from build123d import *

# Parameters (mm, degrees)
SALIENTE_EXTRUIR1_DEPTH    = 2
CROQUIS3_W                 = 28.5
CROQUIS3_H                 = 54
SALIENTE_EXTRUIR2_DEPTH    = 21
CORTAR_EXTRUIR2_DEPTH      = 21
CORTAR_EXTRUIR2_DEPTH_BACK = 61
CORTAR_EXTRUIR2_START      = -23
CROQUIS7_W                 = 26.5
CROQUIS7_H                 = 52
CROQUIS10_W                = 18.5
CROQUIS10_H                = 13
CORTAR_EXTRUIR3_DEPTH      = 10
CROQUIS11_W                = 28.5
CROQUIS11_H                = 54
CORTAR_EXTRUIR4_DEPTH      = 0.9
CROQUIS12_W                = 30
CROQUIS12_H                = 30
CORTAR_EXTRUIR6_DEPTH      = 20.6
CROQUIS13_W                = 3
CROQUIS13_H                = 16
SALIENTE_EXTRUIR5_DEPTH    = 6
SALIENTE_EXTRUIR9_DEPTH    = 16
SALIENTE_EXTRUIR10_DEPTH   = 16
SALIENTE_EXTRUIR11_DEPTH   = 16
SALIENTE_EXTRUIR12_DEPTH   = 16
CROQUIS25_W                = 4.5
CROQUIS25_H                = 1.45
CORTAR_EXTRUIR7_DEPTH      = 0.9
CORTAR_EXTRUIR9_DEPTH      = 0.9
CORTAR_EXTRUIR9_DEPTH_BACK = 1
CROQUIS26_W                = 6
CROQUIS26_H                = 5
CROQUIS32_R                = 2.5
SALIENTE_EXTRUIR13_DEPTH   = 29
CROQUIS36_R                = 1
CORTAR_EXTRUIR10_DEPTH     = 4.5
CROQUIS39_R                = 1
CORTAR_EXTRUIR11_DEPTH     = 4.5
CROQUIS38_R                = 1
CORTAR_EXTRUIR12_DEPTH     = 4.5
CROQUIS37_R                = 1
CORTAR_EXTRUIR13_DEPTH     = 4.5


with BuildPart() as part:
    # Croquis1 → Saliente-Extruir1 (new body)
    with BuildSketch(Plane(origin=(0, 0, 0), x_dir=(1, 0, 0), z_dir=(0, 1, 0))):
        with BuildLine():
            Line((-76.52774776, -47.188914739), (-76.52774776, 21.977990865))
            ThreePointArc((-76.52774776, 21.977990865), (-51.168030611, 47.337708015), (-25.808313462, 21.977990865))
            Line((-25.808313462, 21.977990865), (-25.808313462, -47.033075243))
            ThreePointArc((-25.808313462, -47.033075243), (-51.106035712, -67.287819919), (-76.52774776, -47.188914739))
        make_face()
    extrude(amount=SALIENTE_EXTRUIR1_DEPTH)

    # Croquis3 → Saliente-Extruir2 (add)
    with BuildSketch(Plane(origin=(0, 2, 0), x_dir=(1, 0, 0), z_dir=(0, 1, 0))):
        with Locations((-51.124943413, -32.32840731)):
            Rectangle(CROQUIS3_W, CROQUIS3_H)
    extrude(amount=SALIENTE_EXTRUIR2_DEPTH)

    # Croquis7 → Cortar-Extruir2 (cut, two sides: drawn at the far end of the back side and taken through both)
    with BuildSketch(Plane(origin=(0, 23, 0), x_dir=(1, 0, 0), z_dir=(0, 1, 0)).offset(CORTAR_EXTRUIR2_START - CORTAR_EXTRUIR2_DEPTH_BACK)):
        with Locations((-51.124943413, -32.32840731)):
            Rectangle(CROQUIS7_W, CROQUIS7_H)
    extrude(amount=CORTAR_EXTRUIR2_DEPTH + CORTAR_EXTRUIR2_DEPTH_BACK, mode=Mode.SUBTRACT)

    # Croquis10 → Cortar-Extruir3 (cut)
    with BuildSketch(Plane(origin=(0, 0, 5.32840731), x_dir=(-1, 0, 0), z_dir=(0, 0, -1))):
        with Locations((51.124943413, 8.5)):
            Rectangle(CROQUIS10_W, CROQUIS10_H)
    extrude(amount=-CORTAR_EXTRUIR3_DEPTH, mode=Mode.SUBTRACT)

    # Croquis11 → Cortar-Extruir4 (cut)
    with BuildSketch(Plane.XZ):
        with Locations((-51.124943413, 32.32840731)):
            Rectangle(CROQUIS11_W, CROQUIS11_H)
    extrude(amount=-CORTAR_EXTRUIR4_DEPTH, mode=Mode.SUBTRACT)

    # Croquis12 → Cortar-Extruir6 (cut)
    with BuildSketch(Plane(origin=(0, 2, 0), x_dir=(1, 0, 0), z_dir=(0, 1, 0))):
        with Locations((-51.168030611, 16.67159269)):
            Rectangle(CROQUIS12_W, CROQUIS12_H)
    extrude(amount=-CORTAR_EXTRUIR6_DEPTH, mode=Mode.SUBTRACT)

    # Croquis13 → Saliente-Extruir5 (add)
    with BuildSketch(Plane(origin=(0, 2, 0), x_dir=(1, 0, 0), z_dir=(0, 1, 0))):
        with Locations((-29.308313462, -38.804003852)):
            Rectangle(CROQUIS13_W, CROQUIS13_H)
        with Locations((-73.02774776, -38.95348914)):
            Rectangle(CROQUIS13_W, CROQUIS13_H)
        with Locations((-73.02774776, 13.977990865)):
            Rectangle(CROQUIS13_W, CROQUIS13_H)
        with Locations((-29.308313462, 13.977990865)):
            Rectangle(CROQUIS13_W, CROQUIS13_H)
    extrude(amount=SALIENTE_EXTRUIR5_DEPTH)

    # Croquis18 → Saliente-Extruir9 (add)
    with BuildSketch(Plane.XY.offset(46.804003852)):
        Polygon((-27.808313462, 8), (-27.808313462, 5.3), (-26.608313462, 5.3), align=None)
    extrude(amount=-SALIENTE_EXTRUIR9_DEPTH)

    # Croquis21 → Saliente-Extruir10 (add)
    with BuildSketch(Plane.XY.offset(46.95348914)):
        Polygon((-74.52774776, 8), (-74.52774776, 5.3), (-75.72774776, 5.3), align=None)
    extrude(amount=-SALIENTE_EXTRUIR10_DEPTH)

    # Croquis22 → Saliente-Extruir11 (add)
    with BuildSketch(Plane(origin=(0, 0, -21.977990865), x_dir=(-1, 0, 0), z_dir=(0, 0, -1))):
        Polygon((27.808313462, 8), (27.808313462, 5.3), (26.608313462, 5.3), align=None)
    extrude(amount=-SALIENTE_EXTRUIR11_DEPTH)

    # Croquis23 → Saliente-Extruir12 (add)
    with BuildSketch(Plane(origin=(0, 0, -21.977990865), x_dir=(-1, 0, 0), z_dir=(0, 0, -1))):
        Polygon((74.52774776, 8), (74.52774776, 5.3), (75.72774776, 5.3), align=None)
    extrude(amount=-SALIENTE_EXTRUIR12_DEPTH)

    # Croquis25 → Cortar-Extruir7 (cut)
    with BuildSketch(Plane.XZ):
        with Locations((-53.374943413, 4.60340731)):
            Rectangle(CROQUIS25_W, CROQUIS25_H)
    extrude(amount=-CORTAR_EXTRUIR7_DEPTH, mode=Mode.SUBTRACT)

    # Croquis26 → Cortar-Extruir9 (cut, two sides: drawn at the far end of the back side and taken through both)
    with BuildSketch(Plane(origin=(0, 0, 58.32840731), x_dir=(-1, 0, 0), z_dir=(0, 0, -1)).offset(-CORTAR_EXTRUIR9_DEPTH_BACK)):
        with Locations((55.874943413, 3.4)):
            Rectangle(CROQUIS26_W, CROQUIS26_H)
        with Locations((46.374943413, 3.4)):
            Rectangle(CROQUIS26_W, CROQUIS26_H)
    extrude(amount=CORTAR_EXTRUIR9_DEPTH + CORTAR_EXTRUIR9_DEPTH_BACK, mode=Mode.SUBTRACT)

    # Croquis32 → Saliente-Extruir13 (add)
    with BuildSketch(Plane(origin=(0, 2, 0), x_dir=(1, 0, 0), z_dir=(0, 1, 0))):
        with Locations(Location((-68.12774776, -49.95348914, 0), (0, 0, 90))):
            Circle(CROQUIS32_R)
        with Locations(Location((-68.12774776, -6.95348914, 0), (0, 0, 90))):
            Circle(CROQUIS32_R)
        with Locations(Location((-34.208313462, -50.515469487, 0), (0, 0, 90))):
            Circle(CROQUIS32_R)
        with Locations(Location((-34.208313462, -7.515469487, 0), (0, 0, 90))):
            Circle(CROQUIS32_R)
    extrude(amount=SALIENTE_EXTRUIR13_DEPTH)

    # Croquis36 → Cortar-Extruir10 (cut)
    with BuildSketch(Plane(origin=(0, 31, 0), x_dir=(1, 0, 0), z_dir=(0, 1, 0))):
        with Locations(Location((-68.12774776, -6.95348914, 0), (0, 0, 270))):
            Circle(CROQUIS36_R)
    extrude(amount=-CORTAR_EXTRUIR10_DEPTH, mode=Mode.SUBTRACT)

    # Croquis39 → Cortar-Extruir11 (cut)
    with BuildSketch(Plane(origin=(0, 31, 0), x_dir=(1, 0, 0), z_dir=(0, 1, 0))):
        with Locations(Location((-68.12774776, -49.95348914, 0), (0, 0, 270))):
            Circle(CROQUIS39_R)
    extrude(amount=-CORTAR_EXTRUIR11_DEPTH, mode=Mode.SUBTRACT)

    # Croquis38 → Cortar-Extruir12 (cut)
    with BuildSketch(Plane(origin=(0, 31, 0), x_dir=(1, 0, 0), z_dir=(0, 1, 0))):
        with Locations(Location((-34.208313462, -50.515469487, 0), (0, 0, 270))):
            Circle(CROQUIS38_R)
    extrude(amount=-CORTAR_EXTRUIR12_DEPTH, mode=Mode.SUBTRACT)

    # Croquis37 → Cortar-Extruir13 (cut)
    with BuildSketch(Plane(origin=(0, 31, 0), x_dir=(1, 0, 0), z_dir=(0, 1, 0))):
        with Locations(Location((-34.208313462, -7.515469487, 0), (0, 0, 270))):
            Circle(CROQUIS37_R)
    extrude(amount=-CORTAR_EXTRUIR13_DEPTH, mode=Mode.SUBTRACT)


solid = part.part
Source: CAD feature listing. Evaluate the final solid. Frame: model axes, mm. A direction names the side the tool comes from. Round coordinates to 2 decimals unless told otherwise and drop trailing zeros. Loops run counter-clockwise (first coordinate to the right, second up) from the corner with the lowest first, then second, coordinate; pieces in that order, holes last. Notation, with made-up numbers: M 11.5,38.25 L 40.5,38.25 A34 cw 40.5,74.25 Z; hole C 21.5,-32.5 d4. An arc over 180 degrees is marked long. Return JSON: item names as keys, results as strings. Group by question number.
1. Material intervals for line 1 along X through (y, z) = (10.5, 54.5); line 2 along Z through (x, y) = (-49, 18.5); line 3 along Z through (x, y) = (-50, 1), sorted ascending. Write a range as from..to.
2. Section query C-C on y = 13. Output: boundary loops of the cut face in (x, z).
3. Reachability of faces 4 (the face through (-64.375, 11, 33)), 5 (the face through (-51, 23, 32)), 6 (the face through (-33.251, 16.297, 48.206)) from +Z, -Z, +X, -X, +Y, -Y: full face, straight path, thin tool, end or side. Return the list, or none.
4. Mould query, pull axis X, two halves, no side actions, for faces 1 (the face through (-29, 5, 46.804)), 2 (the face through (-71.528, 5, 39)), 3 (the face through (-74.528, 4, -14)). Classes: released by +X, released by -X, zero draft, split by the parting line, or undercut.
5. Section query D-D on x = -61.5. Output: boundary loops of the cut face in (y, z), and give its area (3 significant figures).
6. Section query A-A on z = -11. Output: boundary loops of the cut face in (x, y).
7. Section query B-B on x = -45.5. Output: boundary loops of the cut face in (y, z).
8. Pin query (flat end, axial travel): pin 1 (5 mm diameter, centred on x = -32.5, y = 9.5, fed in from +Z); pin 2 (10 mm diameter, centred on x = -54, y = 10.5, fed in from +Z); pin 3 (1.8 mm diameter, centred on x = -68.13, z = 49.95, fed in from -Y); pin 4 (1.5 mm diameter, centred on x = -73, z = -10, fed in from +Y). Return the tip coordinate at first contact, or that it passes through.
Checks:
{
 "1": {"line 1": "x = -65.37..-64.37, -37.87..-36.87", "line 2": "z = 5.33..6.33, 58.33..59.33", "line 3": "z = -47.31..-31.67, -1.67..6.33, 58.33..67.26"},
 "2": {"outline": "C -68.13,6.95 d5; C -68.13,49.95 d5; M -65.37,5.33 L -60.37,5.33 L -60.37,6.33 L -64.37,6.33 L -64.37,58.33 L -37.87,58.33 L -37.87,6.33 L -41.87,6.33 L -41.87,5.33 L -36.87,5.33 L -36.87,59.33 L -65.37,59.33 Z; C -34.21,7.52 d5; C -34.21,50.52 d5"},
 "3": {"face 4": "-Y", "face 5": "+Z, -Z, +Y", "face 6": "+Y"},
 "4": {"face 1": "zero draft", "face 2": "undercut", "face 3": "released by -X"},
 "5": {"outline": "M 0,-45.14 L 2,-45.14 L 2,-31.67 L 0,-31.67 Z; M 0,-1.67 L 2,-1.67 L 2,5.33 L 23,5.33 L 23,59.33 L 2,59.33 L 2,65.16 L 0,65.16 L 0,59.33 L 0.9,59.33 L 0.9,58.33 L 21,58.33 L 21,6.33 L 0.9,6.33 L 0.9,5.33 L 0,5.33 Z", "area": "201 mm²"},
 "6": {"outline": "M -76.53,0 L -66.17,0 L -66.17,2 L -71.53,2 L -71.53,8 L -74.53,8 L -75.73,5.3 L -74.53,5.3 L -74.53,2 L -76.53,2 Z; M -36.17,0 L -25.81,0 L -25.81,2 L -27.81,2 L -27.81,5.3 L -26.61,5.3 L -27.81,8 L -30.81,8 L -30.81,2 L -36.17,2 Z"},
 "7": {"outline": "M 0,-46.7 L 2,-46.7 L 2,-31.67 L 0,-31.67 Z; M 0,-1.67 L 2,-1.67 L 2,6.33 L 0.9,6.33 L 0.9,5.33 L 0,5.33 Z; M 0,59.33 L 2,59.33 L 2,66.66 L 0,66.66 Z; M 5.9,58.33 L 21,58.33 L 21,6.33 L 15,6.33 L 15,5.33 L 23,5.33 L 23,59.33 L 5.9,59.33 Z"},
 "8": {"pin 1": "stops at z = 53.02", "pin 2": "stops at z = 59.33", "pin 3": "stops at y = 0", "pin 4": "stops at y = 8"}
}
